from build123d import *

# Parameters (mm, degrees)
BOSS_EXTRUDE1_DEPTH = 20
SKETCH2_R           = 1.75
CUT_EXTRUDE1_DEPTH  = 613.992726316


with BuildPart() as part:
    # Sketch1 → Boss-Extrude1 (new body)
    with BuildSketch(Plane.XY):
        with BuildLine():
            Line((273.434767303, -422.936084161), (270.394702546, -445.835167249))
            Line((270.394702546, -445.835167249), (274.394702546, -446.36620419))
            Line((274.394702546, -446.36620419), (273.067110194, -456.36620419))
            Line((273.067110194, -456.36620419), (261.171482616, -454.78694977))
            add(Edge.make_bspline(
                [(261.171482616, -454.78694977), (296.963881998, -481.467411972), (307.211379584, -530.076645967)],
                knots=[0, 0, 0, 1, 1, 1], degree=2))
            Line((307.211379584, -530.076645967), (306.527614225, -487.761523765))
            Line((306.527614225, -487.761523765), (304.794080931, -380.481047826))
            Line((304.794080931, -380.481047826), (303.947271008, -328.075840548))
            add(Edge.make_bspline(
                [(303.947271008, -328.075840548), (291.93823329, -370.199418032), (265.55288805, -421.8896919)],
                knots=[0, 0, 0, 1, 1, 1], degree=2))
            Line((265.55288805, -421.8896919), (273.434767303, -422.936084161))
        make_face()
    extrude(amount=BOSS_EXTRUDE1_DEPTH)

    # Sketch2 → Cut-Extrude1 (cut, through all)
    with BuildSketch(Plane.XY.offset(20)):
        with Locations((288.352935212, -464.179893051)):
            Circle(SKETCH2_R)
        with Locations((290.016681941, -451.647832837)):
            Circle(SKETCH2_R)
        with Locations((291.68042867, -439.115772622)):
            Circle(SKETCH2_R)
    extrude(amount=-CUT_EXTRUDE1_DEPTH, mode=Mode.SUBTRACT)


solid = part.part
Check sheet for the modelled part. Datum: model origin and axes. Units: mm. A direction names the side the tool comes from. Round coordinates to 2 decimals unless told otherwise and drop trailing zeros.
(1) Cross-section at A-A, the plane z = 4. State how many separate pieces and enclosed holes the cut face has, and give its area (3 significant figures).
(2) Go/stop test with flat-tipped pins: P1, Ø12, axis at x = 272.5, z = 12, coming from the +Y side; P2, Ø6, axis at y = -437, z = 10, coming from the -X side; P3, Ø5, axis at y = -386, z = 4.5, coming from the +X side; P4, Ø4, axis at x = 293.5, y = -369.5, coming from the -Z side. Record where each tip stops, or that it passes through.
(3) Scan lines: probe 1 along Y at (x, z) = (269.5, 4.5); probe 2 along X at (y, z) = (-453, 9); probe 3 along X at (y, z) = (-505, 4). Record each from-to range of solid material in increasing order.
(4) Access from +Z, -Z, +X, -X, +Y, -Y to the whole of each face (thin tool, end or side, straight path). Record for faces 1 (the flat face through (267.203, -455.588, 9.86)), 2 (the flat face through (271.936, -434.225, 9.86)), 3 (the flat face through (294, -428, 20)).
(5) Draft check along X on faces 4 (the flat face through (272.4, -446.1, 9.9)), 5 (the cylindrical face through (288.125, -462.445, 10.14)), 6 (the flat face through (294, -428, 0)). Enter one of: pulls with the +X half, pulls with the -X half, needs draft (parallel to the pull), parting line crosses it, or undercut.
Check sheet entries:
1. separate pieces: 1
1. enclosed holes: 3
1. area: 3,970 mm2
2. P1: stops at y = -395.23
2. P2: stops at x = 271.17
2. P3: stops at x = 304.92
2. P4: stops at z = 0
3. probe 1: y = -461.6 to -455.89, -422.41 to -414.05
3. probe 2: x = 273.51 to 288.91, 291.13 to 305.97
3. probe 3: x = 299.64 to 306.81
4. face 1: +Z, -Z
4. face 2: +Z, -Z, -X
4. face 3: +Z, +X, -X, +Y, -Y
5. face 4: pulls with the -X half
5. face 5: undercut
5. face 6: needs draft
